from build123d import *

# Parameters (mm, degrees)
BOSS_EXTRUDE1_DEPTH     = 3.571875
SKETCH2_W               = 45
SKETCH2_H               = 3.571875
BOSS_EXTRUDE2_DEPTH     = 19.05
FILLET1_R               = 2
SKETCH9_W               = 44.9012818
SKETCH9_H               = 1.417156311
CUT_EXTRUDE1_DEPTH      = 10
BOSS_EXTRUDE3_DEPTH     = 3.571875
SKETCH14_R              = 1.8034
CUT_EXTRUDE4_DEPTH      = 4.571875
FILLET3_R               = 2.54
SKETCH15_R              = 6.75
SKETCH15_R_2            = 1.55
CUT_EXTRUDE5_DEPTH      = 21.367363974
CUT_EXTRUDE5_DEPTH_BACK = 4.571875


with BuildPart() as part:
    # Sketch1 → Boss-Extrude1 (new body)
    with BuildSketch(Plane.XY.offset(5)):
        with BuildLine():
            Line((-21.183407813, 0), (-21.183407813, -8.813455393))
            ThreePointArc((-21.183407813, -8.813455393), (-22.866221682, -12.686440931), (-19.530849883, -15.276262248))
            Line((-19.530849883, -15.276262248), (24.68248716, -15.276262248))
            ThreePointArc((24.68248716, -15.276262248), (25.214329472, -14.744419936), (24.68248716, -14.212577623))
            Line((24.68248716, -14.212577623), (23.717873987, 0))
            Line((23.717873987, 0), (23.717873987, 4.989031311))
            Line((23.717873987, 4.989031311), (-21.183407813, 4.989031311))
            Line((-21.183407813, 4.989031311), (-21.183407813, 0))
        make_face()
    extrude(amount=-BOSS_EXTRUDE1_DEPTH)

    # Sketch2 → Boss-Extrude2 (add)
    with BuildSketch(Plane.XY.offset(5)):
        with Locations((1.270019176, 1.7859375)):
            Rectangle(SKETCH2_W, SKETCH2_H)
    extrude(amount=BOSS_EXTRUDE2_DEPTH)

    # Fillet1
    fillet1_edges = [part.edges().sort_by_distance(p)[0] for p in [
        (1.267233087, 4.989031311, 1.428125),
    ]]
    fillet(fillet1_edges, radius=FILLET1_R)

    # Sketch9 → Cut-Extrude1 (cut)
    with BuildSketch(Plane.XY.offset(5)):
        with Locations((1.267233087, 4.280453156)):
            Rectangle(SKETCH9_W, SKETCH9_H)
    extrude(amount=-CUT_EXTRUDE1_DEPTH, mode=Mode.SUBTRACT)

    # Sketch13 → Boss-Extrude3 (add, through all)
    with BuildSketch(Plane.XY.offset(5)):
        Polygon((-21.229980824, 3.571875), (-39.190493066, -14.388637242), (-39.190493066, -20.367363974), (41.730531418, -20.367363974), (41.730531418, -14.388637242), (23.770019176, 3.571875), align=None)
    extrude(amount=-BOSS_EXTRUDE3_DEPTH)

    # Sketch14 → Cut-Extrude4 (cut, through all)
    with BuildSketch(Plane.XY.offset(5)):
        with Locations((-28.755435454, -14.729886975)):
            Circle(SKETCH14_R)
        with Locations((-20.888731092, -6.863182613)):
            Circle(SKETCH14_R)
        with Locations((23.428769443, -6.863182613)):
            Circle(SKETCH14_R)
        with Locations((31.295473805, -14.729886975)):
            Circle(SKETCH14_R)
    extrude(amount=-CUT_EXTRUDE4_DEPTH, mode=Mode.SUBTRACT)

    # Fillet3
    fillet3_edges = [part.edges().sort_by_distance(p)[0] for p in [
        (23.770019176, 1.7859375, 5),
        (-21.229980824, 1.7859375, 5),
        (23.770019176, 1.7859375, 24.05),
        (-21.229980824, 1.7859375, 24.05),
        (41.730531418, -20.367363974, 3.2140625),
        (-39.190493066, -20.367363974, 3.2140625),
        (-39.190493066, -14.388637242, 3.2140625),
        (41.730531418, -14.388637242, 3.2140625),
    ]]
    fillet(fillet3_edges, radius=FILLET3_R)

    # Sketch15 → Cut-Extrude5 (cut, two sides)
    with BuildSketch(Plane.XZ) as cut_extrude5_sk:
        with Locations((1.270019176, 15.652125)):
            Circle(SKETCH15_R)
        with Locations((-7.729980824, 24.652125)):
            Circle(SKETCH15_R_2)
        with Locations((10.270019176, 24.652125)):
            Circle(SKETCH15_R_2)
    extrude(amount=CUT_EXTRUDE5_DEPTH, mode=Mode.SUBTRACT)
    extrude(cut_extrude5_sk.sketch, amount=-CUT_EXTRUDE5_DEPTH_BACK, mode=Mode.SUBTRACT)


solid = part.part
Can you work these out from the model? Positions are in its coordinate system, mm. A direction names the side the tool comes from. Coordinates: 2 decimals unless noted, no trailing zeros. Write each loop counter-clockwise with the first axis right and the second up, starting at its lowest first coordinate (ties: lowest second). Pieces come first, ordered by that corner, then holes.
Q1. If we mould it in two halves opening along X, with no side actions, what happens to faces 1 (the face through (0.391, 1.761, 22.345)), 2 (the face through (-14, 2, 24.05)), 3 (the face through (24.246, 1.414, 6.06))? For each: +X half, -X half, draft (parallel to the pull), parting line (faces both ways), or undercut.
Results found:
face 1: undercut
face 2: draft
face 3: +X half
Q2. For P1, Ø4, axis at x = 5, z = 9.5, coming from the -Y side; P2, Ø6, axis at y = -1.5, z = 10.5, coming from the +X side; P3, Ø12, axis at x = -29.5, y = -11, coming from the +Z side, each with a flat end and sliding along its axis, tell me the tip position at first contact or that it passes through.
Results found:
P1: stops at y = 0
P2: stops at x = 23.77
P3: stops at z = 5
Q3. Imagine slicing it at D-D, the plane x = 17. List the corners of the cut face in (y, z) for me.
Results found:
outline: (-20.37, 1.43) - (3.57, 1.43) - (3.57, 24.05) - (0, 24.05) - (0, 5) - (-20.37, 5) - close
Q4. Imagine slicing it at C-C, the plane z = 4. List the corners of the cut face in (x, y) for me.
Results found:
outline: (-39.19, -17.83) arc R2.54 ccw to (-36.65, -20.37) - (39.19, -20.37) arc R2.54 ccw to (41.73, -17.83) - (41.73, -15.44) arc R2.54 ccw to (40.99, -13.64) - (23.77, 3.57) - (-21.23, 3.57) - (-38.45, -13.64) arc R2.54 ccw to (-39.19, -15.44) - close; hole circle Ø3.61 at (-28.76, -14.73); hole circle Ø3.61 at (-20.89, -6.86); hole circle Ø3.61 at (23.43, -6.86); hole circle Ø3.61 at (31.3, -14.73)
Q5. Which directions (+Z, -Z, +X, -X, +Y, -Y) give clear straight access to the entire face, cutting with the end or side of a thin tool? Please do faces 4 (the face through (-7.755, 1.761, 23.102)), 5 (the face through (6, 0, 10)), 6 (the face through (-21.23, 2, 14)).
Results found:
face 4: +Z, +Y, -Y
face 5: +Z, +X, -X, -Y
face 6: +Z, -X, +Y, -Y
Q6. Please list where these lines run through material, in increasing order: L1, parallel to Z at x = 26.5, y = -15; L2, parallel to X at y = 2.5, z = 12.5; L3, parallel to Y at x = 11, z = 5.75.
Results found:
L1: z = 1.43 to 5
L2: x = -21.23 to -4.7, 7.24 to 23.77
L3: y = 0 to 3.57
Q7. Imagine slicing it at B-B, the plane y = 1.75. List the corners of the cut face in (x, z) for me, plus the area to 3 significant figures.
Results found:
outline: (-23.05, 1.43) - (25.59, 1.43) - (25.59, 5.1) arc R2.54 cw to (23.77, 7.54) - (23.77, 21.51) arc R2.54 ccw to (21.23, 24.05) - (11.7, 24.05) arc R1.55 cw to (8.84, 24.05) - (-6.3, 24.05) arc R1.55 cw to (-9.16, 24.05) - (-18.69, 24.05) arc R2.54 ccw to (-21.23, 21.51) - (-21.23, 7.54) arc R2.54 cw to (-23.05, 5.1) - close; hole circle Ø13.5 at (1.27, 15.65)
area: 884 mm2
Q8. Imagine slicing it at A-A, the plane x = 6.5. List the corners of the cut face in (y, z) for me, plus the area to 3 significant figures.
Results found:
outline: (-20.37, 1.43) - (3.57, 1.43) - (3.57, 11.38) - (0, 11.38) - (0, 5) - (-20.37, 5) - close; (0, 19.92) - (3.57, 19.92) - (3.57, 24.05) - (0, 24.05) - close
area: 123 mm2
